Here's the drawing with two shaded views (mm, measured from the low corner). I have some questions. Give positions to 0.01 mm unless a question says otherwise; leave off trailing zeros. Write each loop counter-clockwise with the first axis right and the second up, starting at its lowest first coordinate (ties: lowest second). Pieces come first, ordered by that corner, then holes. Notation, with made-up numbers: M -3.75,40 L 25.25,40 A29 cw 25.25,68 Z; hole C 85,-19 d8. An arc over 180 degrees is marked long. Use one line per item in the form item = value.
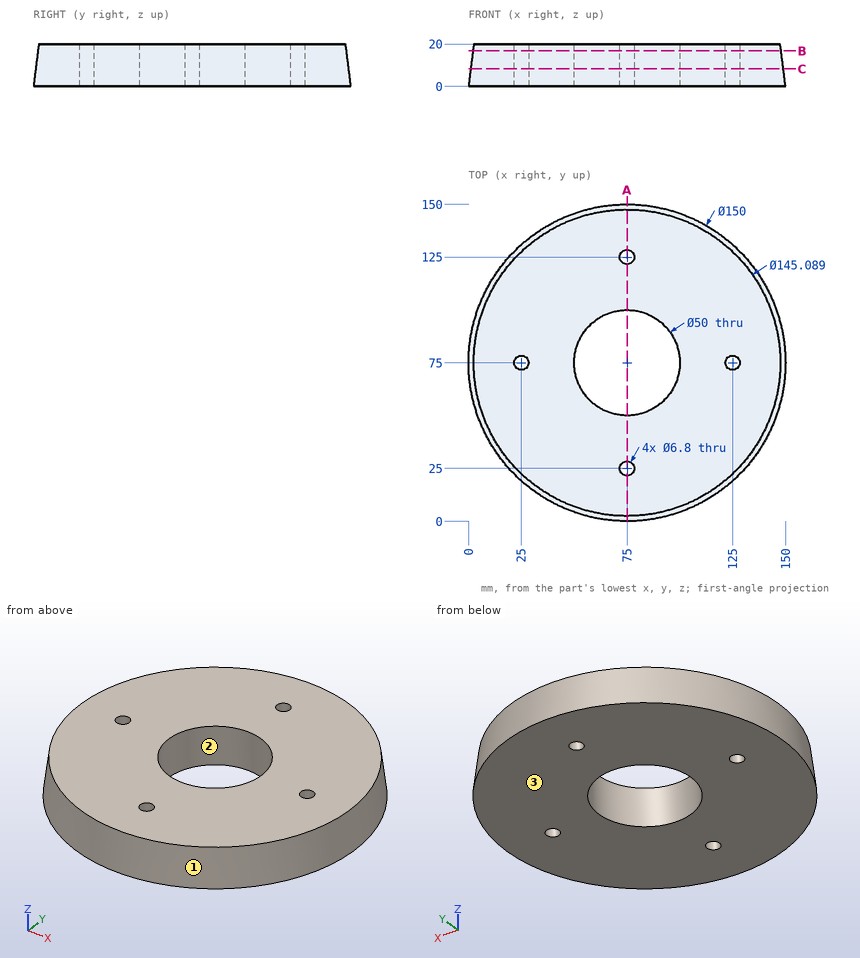
1) I want a section at A-A, the plane x = 75. Please give me the cut outline in (y, z) (1 decimal).
Checked values:
outline = M 0,0 L 21.6,0 L 21.6,20 L 2.5,20 Z; M 28.4,0 L 50,0 L 50,20 L 28.4,20 Z; M 100,0 L 121.6,0 L 121.6,20 L 100,20 Z; M 128.4,0 L 150,0 L 147.5,20 L 128.4,20 Z
2) Thinking about a two-plate mould opening in Y: for the marked faces 1, 2 and 3, which applies, released by +Y, released by -Y, zero draft, split by the parting line, or undercut?
Checked values:
face_1 = split by the parting line
face_2 = undercut
face_3 = zero draft
3) If I drill on L1, parallel to Y at x = 75, z = 5; L2, parallel to Y at x = 75, z = 11; L3, parallel to X at y = 98, z = 10.5 (1 decimal), over which ranges is the centre line in solid material (lowest first)?
Checked values:
L1 = 0.61 to 21.6, 28.4 to 50, 100 to 121.6, 128.4 to 149.39
L2 = 1.35 to 21.6, 28.4 to 50, 100 to 121.6, 128.4 to 148.65
L3 = 5 to 65.2, 84.8 to 145
4) For pin 1 Ø10 at (x, z) = (23, 3.5) entering from -Y; pin 2 Ø8 at (x, z) = (23.5, 14.5) entering from -Y; pin 3 Ø1 at (x, z) = (25.5, 16.5) entering from -Y, each with a flat end and sliding along its axis, tell me the tip position at first contact or that it passes through.
Checked values:
pin_1 = 17.03
pin_2 = 19.22
pin_3 = 20.92
5) I want a section at B-B, the plane z = 16.75. Please give me the cut outline in (x, y), plus the area to 3 significant figures.
Checked values:
outline = C 75,75 d145.89; hole C 25,75 d6.8; hole C 75,75 d50; hole C 75,25 d6.8; hole C 75,125 d6.8; hole C 125,75 d6.8
area = 14,600 mm2
6) I want a section at C-C, the plane z = 8.25. Please give me the cut outline in (x, y), plus the area to 3 significant figures.
Checked values:
outline = C 75,75 d147.97; hole C 25,75 d6.8; hole C 75,75 d50; hole C 75,25 d6.8; hole C 75,125 d6.8; hole C 125,75 d6.8
area = 15,100 mm2
